from build123d import *

# Parameters (mm, degrees)
F2_DEPTH = 3.5
F3_R     = 1.5875
F4_DEPTH = 6


with BuildPart() as f2:
    # F1 (on Front) → F2 (new body, symmetric)
    with BuildSketch(Plane.XZ):
        Polygon((1.5875, -4), (1.5875, 0), (-1.5875, 0), (-1.5875, -4), (-5.25, -4), (-5.25, -11.5), (5.25, -11.5), (5.25, -4), align=None)
    extrude(amount=F2_DEPTH, both=True)

    # F3 (on Top) → F4 (join)
    with BuildSketch(Plane.XY):
        Circle(F3_R)
    extrude(amount=F4_DEPTH)


solid = f2.part
For this review, take the finished solid that the model builds, in its own axes (mm). A direction names the side the tool comes from. Coordinates: 2 decimals unless noted, no trailing zeros. Write each loop counter-clockwise with the first axis right and the second up, starting at its lowest first coordinate (ties: lowest second). Pieces come first, ordered by that corner, then holes. Notation, with made-up numbers: (6.5, 1) -> (10.5, 1) arc R20 cw to (10.5, 38) -> close; hole circle Ø7 at (-28.75, 20). An arc over 180 degrees is marked (long way). Write each question's results on one line, items separated by ' | '. Start each with the question number.
1) Consider section B-B (x = 0). Write out the cut boundary in (y, z).
2) Consider section C-C (z = 3). Write out the cut boundary in (x, y) (1 decimal).
3) Insertion check: pin 1 (6 mm diameter, centred on x = 1, z = 4, fed in from +Y); pin 2 (1.5 mm diameter, centred on y = -1.5, z = 2, fed in from +X); pin 3 (3 mm diameter, centred on x = -2.5, z = -2.5, fed in from +Y); pin 4 (1.1 mm diameter, centred on x = -3.5, y = 1, fed in from +Z). Each pin has a flat end and moves straight along its axis. Give the tip position at first contact, or say it passes through.
4) Consider section D-D (x = 4.75). Write out the cut boundary in (y, z).
5) Wall thickness on L1, parallel to Z at x = -2.5, y = -3; L2, parallel to X at y = 3.25, z = -0.75; L3, parallel to Z at x = 1.25, y = 1.25: over which ranges is each line inside the solid? List them lowest first. Write a range as [from, to].
6) For faces 1 (the face through (3, 0, -4)), 2 (the face through (0, 3.5, -7)), 3 (the face through (-0.34, -1.55, 2.96)), 4 (the face through (-1.588, 0, -2)), list the 3-axis set-ups (+Z, -Z, +X, -X, +Y, -Y) from which the entire face can be reached by the end or side of a thin tool; tool diameter is ignored.
7) Consider section A-A (y = 3.25). Write out the cut boundary in (x, z).
Geometry says:
1) outline: (-3.5, -11.5) -> (3.5, -11.5) -> (3.5, 0) -> (1.59, 0) -> (1.59, 6) -> (-1.59, 6) -> (-1.59, 0) -> (-3.5, 0) -> close
2) outline: circle Ø3.2 at (0, 0)
3) pin 1: y = 1.59 | pin 2: x = 1.4 | pin 3: y = 3.5 | pin 4: z = -4
4) outline: (-3.5, -11.5) -> (3.5, -11.5) -> (3.5, -4) -> (-3.5, -4) -> close
5) L1: [-11.5, -4] | L2: [-1.59, 1.59] | L3: [-11.5, 0]
6) face 1: +Z, +X, +Y, -Y | face 2: +Z, -Z, +X, -X, +Y | face 3: +Z | face 4: +Z, -X, +Y, -Y
7) outline: (-5.25, -11.5) -> (5.25, -11.5) -> (5.25, -4) -> (1.59, -4) -> (1.59, 0) -> (-1.59, 0) -> (-1.59, -4) -> (-5.25, -4) -> close
